Geometry: see drawing. Coordinates: mm, zero at the bounding-box minimum. Give positions to 0.01 mm unless a question says otherwise; leave off trailing zeros. Write each loop counter-clockwise with the first axis right and the second up, starting at its lowest first coordinate (ties: lowest second). Pieces come first, ordered by that corner, then holes. Notation, with made-up numbers: (15.25, 34) -> (23.25, 34) arc R18 ccw to (23.25, 59) -> close; hole circle Ø1 at (79.25, 57). An arc over 180 degrees is marked (long way). Write item = value, one per line.
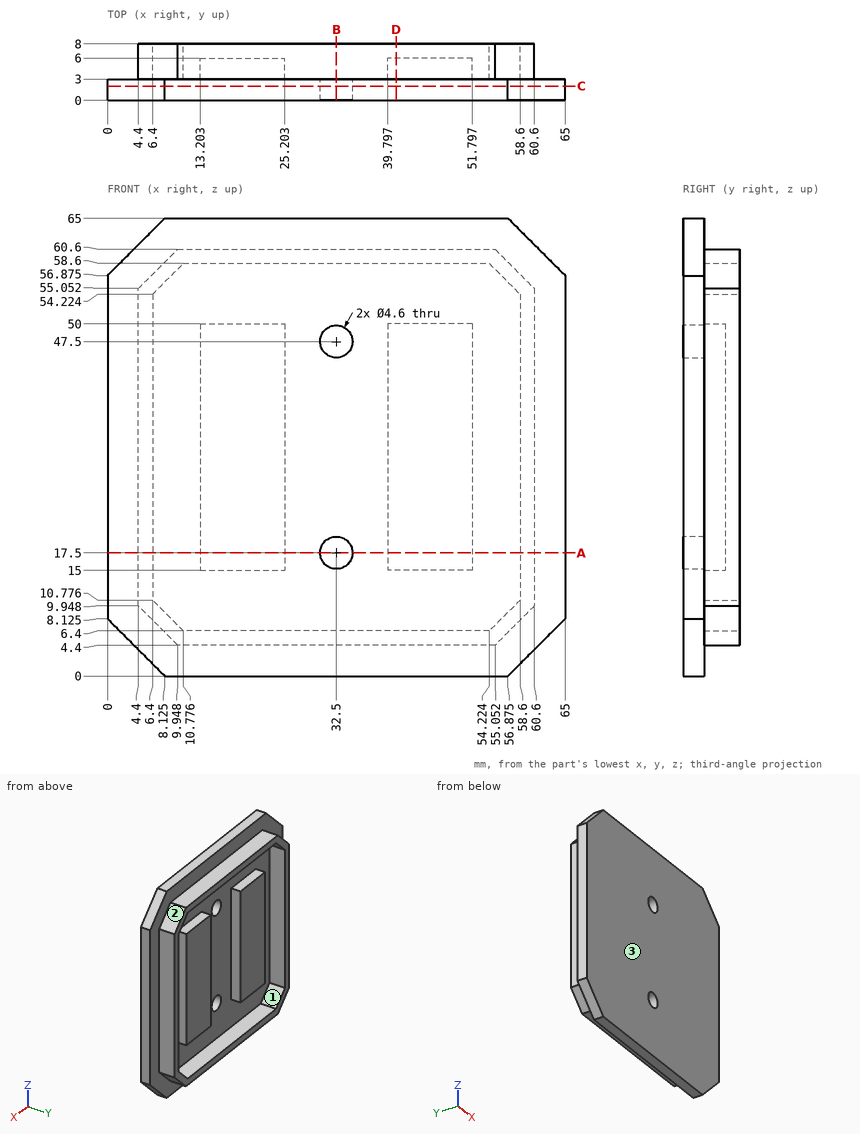
(1) First-contact query: pin 1 (2.5 mm diameter, centred on x = 43, y = 4, fed in from +Z); pin 2 (4 mm diameter, centred on x = 32.5, z = 17.5, fed in from -Y); pin 3 (4 mm diameter, centred on y = 6, z = 28, fed in from -X); pin 4 (2.5 mm diameter, centred on y = 4.5, z = 29, fed in from +X). Flat tips, straight axial feed; report the tip coordinate or a pass-through.
Values follow:
pin_1 = 65
pin_2 = through
pin_3 = 4.4
pin_4 = 60.6
(2) Section query D-D (x = 41). Return loops of the section in (y, z).
Values follow:
outline = (0, 0) -> (3, 0) -> (3, 4.4) -> (8, 4.4) -> (8, 6.4) -> (3, 6.4) -> (3, 15) -> (6, 15) -> (6, 50) -> (3, 50) -> (3, 58.6) -> (8, 58.6) -> (8, 60.6) -> (3, 60.6) -> (3, 65) -> (0, 65) -> close
(3) Material intervals for line 1 (Z direction, x = 25, y = 3.75); line 2 (Z direction, x = 36.5, y = 6); line 3 (X direction, y = 2.25, z = 17.5), sorted ascending.
Values follow:
line_1 = 4.4 to 6.4, 15 to 50, 58.6 to 60.6
line_2 = 4.4 to 6.4, 58.6 to 60.6
line_3 = 0 to 30.2, 34.8 to 65
(4) Section query C-C (y = 2). Return loops of the section in (x, z) (1 decimal).
Values follow:
outline = (0, 8.1) -> (8.1, 0) -> (56.9, 0) -> (65, 8.1) -> (65, 56.9) -> (56.9, 65) -> (8.1, 65) -> (0, 56.9) -> close; hole circle Ø4.6 at (32.5, 17.5); hole circle Ø4.6 at (32.5, 47.5)
(5) Section query B-B (x = 32.5). Return loops of the section in (y, z).
Values follow:
outline = (0, 0) -> (3, 0) -> (3, 4.4) -> (8, 4.4) -> (8, 6.4) -> (3, 6.4) -> (3, 15.2) -> (0, 15.2) -> close; (0, 19.8) -> (3, 19.8) -> (3, 45.2) -> (0, 45.2) -> close; (0, 49.8) -> (3, 49.8) -> (3, 58.6) -> (8, 58.6) -> (8, 60.6) -> (3, 60.6) -> (3, 65) -> (0, 65) -> close
(6) Pull-direction query (Z, two-part tool) for the marked faces 1, 2 and 3; classes: pulls with the +Z half, pulls with the -Z half, needs draft (parallel to the pull), parting line crosses it, or undercut.
Values follow:
face_1 = undercut
face_2 = pulls with the +Z half
face_3 = needs draft
(7) Section query A-A (z = 17.5). Return loops of the section in (x, y), plus the area to 3 significant figures.
Values follow:
outline = (0, 0) -> (30.2, 0) -> (30.2, 3) -> (25.2, 3) -> (25.2, 6) -> (13.2, 6) -> (13.2, 3) -> (6.4, 3) -> (6.4, 8) -> (4.4, 8) -> (4.4, 3) -> (0, 3) -> close; (34.8, 0) -> (65, 0) -> (65, 3) -> (60.6, 3) -> (60.6, 8) -> (58.6, 8) -> (58.6, 3) -> (51.8, 3) -> (51.8, 6) -> (39.8, 6) -> (39.8, 3) -> (34.8, 3) -> close
area = 273 mm2
